CAD build for the part. Positions are in the model's coordinates, mm. A direction names the side the tool comes from. Round coordinates to 2 decimals unless told otherwise and drop trailing zeros. Write each loop counter-clockwise with the first axis right and the second up, starting at its lowest first coordinate (ties: lowest second). Pieces come first, ordered by that corner, then holes. Notation, with made-up numbers: (-16, 7) -> (-6, 7) arc R34 ccw to (-6, 45) -> close; hole circle Ø10 at (29.5, -3). An arc over 180 degrees is marked (long way). Put each result on its own line as item: value. Start each with the question number.
1. Drill centre lines: line 1 (Y direction, x = 5.25, z = -25.4) (3 decimals); line 2 (Z direction, x = 5, y = -97); line 3 (Y direction, x = 2.25, z = -60.5). Where is each one in solid material? Low to high. Write a range as from..to.
2. Saw through at B-B on y = -105.5. List the corners of the cut face in (x, z), and give its area (3 significant figures).
3. 3-axis set-ups, long thin cutter, end or side, ignore diameter. For faces 1 (the cylindrical face through (3.091, -126.206, 6.298)), 2 (the flat face through (3, 12.7, -88)): which of +Z, -Z, +X, -X, +Y, -Y reach the whole face in a straight line?
4. Saw through at D-D on x = 4.25. State how many separate pieces and enclosed holes the cut face has, and give its area (3 significant figures).
5. Saw through at A-A on z = -127. List the corners of the cut face in (x, y) (3 decimals), and give its area (3 significant figures).
6. Saw through at C-C on y = -179. List the corners of the cut face in (x, z).
from build123d import *

# Parameters (mm, degrees)
SKETCH1_W               = 203.2
SKETCH1_H               = 222.25
SKETCH1_R               = 2.425
SKETCH1_W_2             = 177.8
SKETCH1_H_2             = 184.15
BOSS_EXTRUDE1_DEPTH     = 6.096
FILLET1_R               = 2.54
CUT_EXTRUDE1_DEPTH      = 7.096
SKETCH3_R               = 2.505
CUT_EXTRUDE2_DEPTH      = 1
CUT_EXTRUDE2_DEPTH_BACK = 7.096


with BuildPart() as part:
    # Sketch1 → Boss-Extrude1 (new body)
    with BuildSketch(Plane(origin=(0, 0, 0), x_dir=(0, 0, -1), z_dir=(1, 0, 0))):
        with Locations((88.9, -98.425)):
            Rectangle(SKETCH1_W, SKETCH1_H)
        with Locations((0, -196.85)):
            Circle(SKETCH1_R, mode=Mode.SUBTRACT)
        with Locations((25.4, -196.85)):
            Circle(SKETCH1_R, mode=Mode.SUBTRACT)
        with Locations((50.8, -196.85)):
            Circle(SKETCH1_R, mode=Mode.SUBTRACT)
        with Locations((76.2, -196.85)):
            Circle(SKETCH1_R, mode=Mode.SUBTRACT)
        with Locations((101.6, -196.85)):
            Circle(SKETCH1_R, mode=Mode.SUBTRACT)
        with Locations((127, -196.85)):
            Circle(SKETCH1_R, mode=Mode.SUBTRACT)
        with Locations((152.4, -196.85)):
            Circle(SKETCH1_R, mode=Mode.SUBTRACT)
        with Locations((177.8, -196.85)):
            Circle(SKETCH1_R, mode=Mode.SUBTRACT)
        with Locations((88.9, -92.075)):
            Rectangle(SKETCH1_W_2, SKETCH1_H_2, mode=Mode.SUBTRACT)
    extrude(amount=BOSS_EXTRUDE1_DEPTH)

    # Fillet1
    fillet1_edges = [part.edges().sort_by_distance(p)[0] for p in [
        (3.048, 0, 0),
        (3.048, -184.15, 0),
        (3.048, -184.15, -177.8),
        (3.048, 0, -177.8),
        (3.048, 12.7, 12.7),
        (3.048, 12.7, -190.5),
        (3.048, -209.55, -190.5),
        (3.048, -209.55, 12.7),
    ]]
    fillet(fillet1_edges, radius=FILLET1_R)

    # Sketch2 → Cut-Extrude1 (cut, through all)
    with BuildSketch(Plane(origin=(6.096, 0, 0), x_dir=(0, 0, -1), z_dir=(1, 0, 0))):
        with BuildLine():
            Line((-3.96875, -60.325), (-3.96875, -123.825))
            ThreePointArc((-3.96875, -123.825), (-6.35, -126.20625), (-8.73125, -123.825))
            Line((-8.73125, -123.825), (-8.73125, -60.325))
            ThreePointArc((-8.73125, -60.325), (-6.35, -57.94375), (-3.96875, -60.325))
        make_face()
        with BuildLine():
            Line((181.76875, -60.325), (181.76875, -123.825))
            ThreePointArc((181.76875, -123.825), (184.15, -126.20625), (186.53125, -123.825))
            Line((186.53125, -123.825), (186.53125, -60.325))
            ThreePointArc((186.53125, -60.325), (184.15, -57.94375), (181.76875, -60.325))
        make_face()
    extrude(amount=-CUT_EXTRUDE1_DEPTH, mode=Mode.SUBTRACT)

    # Sketch3 → Cut-Extrude2 (cut, two sides)
    with BuildSketch(Plane(origin=(6.096, 0, 0), x_dir=(0, 0, -1), z_dir=(1, 0, 0))) as cut_extrude2_sk:
        with Locations((177.8, 6.35)):
            Circle(SKETCH3_R)
        with Locations((0, 6.35)):
            Circle(SKETCH3_R)
    extrude(amount=CUT_EXTRUDE2_DEPTH, mode=Mode.SUBTRACT)
    extrude(cut_extrude2_sk.sketch, amount=-CUT_EXTRUDE2_DEPTH_BACK, mode=Mode.SUBTRACT)


solid = part.part
Return value:
1. line 1: y = -209.55..-199.275, -194.425..-184.15, 0..12.7
1. line 2: z = -190.5..-186.53, -181.77..-177.8, 0..3.97, 8.73..12.7
1. line 3: y = -209.55..-184.15, 0..12.7
2. outline: (0, -190.5) -> (6.1, -190.5) -> (6.1, -186.53) -> (0, -186.53) -> close; (0, -181.77) -> (6.1, -181.77) -> (6.1, -177.8) -> (0, -177.8) -> close; (0, 0) -> (6.1, 0) -> (6.1, 3.97) -> (0, 3.97) -> close; (0, 8.73) -> (6.1, 8.73) -> (6.1, 12.7) -> (0, 12.7) -> close
2. area: 96.8 mm^2
3. face 1: +X, -X
3. face 2: +Z, -Z, +X, -X, +Y
4. separate pieces: 1
4. enclosed holes: 13
4. area: 11,600 mm^2
5. outline: (0, -209.55) -> (6.096, -209.55) -> (6.096, -199.275) -> (0, -199.275) -> close; (0, -194.425) -> (6.096, -194.425) -> (6.096, -184.15) -> (0, -184.15) -> close; (0, 0) -> (6.096, 0) -> (6.096, 12.7) -> (0, 12.7) -> close
5. area: 203 mm^2
6. outline: (0, -190.5) -> (6.1, -190.5) -> (6.1, -177.8) -> (0, -177.8) -> close; (0, 0) -> (6.1, 0) -> (6.1, 12.7) -> (0, 12.7) -> close
